Here's how the part is built. I have some questions about the finished solid (model axes, mm). A direction names the side the tool comes from. Give positions to 0.01 mm unless a question says otherwise; leave off trailing zeros. Loops run counter-clockwise (first coordinate to the right, second up) from the corner with the lowest first, then second, coordinate; pieces in that order, holes last. Notation, with made-up numbers: (87.25, 67.25) - (145.25, 67.25) arc R22 ccw to (145.25, 105.25) - close; hole circle Ø6 at (30.5, 54). An arc over 180 degrees is marked (long way). Return JSON: item names as keys, results as strings. Group by question number.
(1) I need wall thicknesses on probe 1 along Y at (x, z) = (50, 2.5); probe 2 along X at (y, z) = (-33, 29); probe 3 along Y at (x, z) = (-183.5, 14.5). Which ranges of each line are inside material? Lowest first, please. Write a range as [from, to].
(2) If we section it at D-D (z = 39.5): State how many separate pieces and enclosed holes the cut face has, then the cut area to 3 significant figures.
(3) If we mould it in two halves opening along X, with no side actions, what happens to faces 1 (the flat face through (204.032, 79, 25)), 2 (the flat face through (-227.768, 30, 25)), 3 (the flat face through (115, 0, 25)), 4 (the flat face through (-2, 81, 0))? For each: released by +X, released by -X, zero draft, split by the parting line, or undercut.
(4) If we section it at A-A (y = -40.5): Please give me the cut outline in (x, z), then the cut area to 3 significant figures.
(5) On a 3-axis mill with a long thin cutter (end or side, diameter ignored), from which of +Z, -Z, +X, -X, +Y, -Y can I reach the whole of each face in a straight line? I mean faces 5 (the flat face through (-2, -201.924, 25)), 6 (the flat face through (-202.368, 78, 25)). Say none if no direction works.
(6) If we section it at B-B (x = 93): Please give me the cut outline in (y, z).
(7) If we section it at C-C (y = 188): Please give me the cut outline in (x, z), then the cut area to 3 significant figures.
```python
from build123d import *

# Parameters (mm, degrees)
F1_DEPTH = 50.8
F2_DEPTH = 50.8
F3_DEPTH = 50.8
F0_W     = 53.3528286101
F0_H     = 176.523585695
F0_W_2   = 176.523585695
F0_H_2   = 53.3528286101
F4_DEPTH = 50.8


with BuildPart() as f1:
    # F0 (on Top) → F1 (new body)
    with BuildSketch(Plane.XY):
        Polygon((-202.3678548309, 229.876414305), (-227.7678548309, 255.276414305), (-227.7678548309, -201.923585695), (-202.3678548309, -176.523585695), (-202.3678548309, -104.6815367264), (-202.3678548309, -50.8), (-202.3678548309, 0), (-202.3678548309, 53.3528286101), (-202.3678548309, 104.1528286101), (-202.3678548309, 158.0343653365), align=None)
        Polygon((-202.3678548309, -176.523585695), (-227.7678548309, -201.923585695), (229.4321451691, -201.923585695), (204.0321451691, -176.523585695), (132.1900962006, -176.523585695), (78.3085594741, -176.523585695), (27.5085594741, -176.523585695), (-25.8442691359, -176.523585695), (-76.6442691359, -176.523585695), (-130.5258058623, -176.523585695), align=None)
        Polygon((229.4321451691, -201.923585695), (229.4321451691, 255.276414305), (204.0321451691, 229.876414305), (204.0321451691, 158.0343653365), (204.0321451691, 104.1528286101), (204.0321451691, 53.3528286101), (204.0321451691, 0), (204.0321451691, -50.8), (204.0321451691, -104.6815367264), (204.0321451691, -176.523585695), align=None)
        Polygon((229.4321451691, 255.276414305), (-227.7678548309, 255.276414305), (-202.3678548309, 229.876414305), (-130.5258058623, 229.876414305), (-76.6442691359, 229.876414305), (-25.8442691359, 229.876414305), (27.5085594741, 229.876414305), (78.3085594741, 229.876414305), (132.1900962006, 229.876414305), (204.0321451691, 229.876414305), align=None)
    extrude(amount=F1_DEPTH)

    # F0 (on Top) → F2 (cut)
    with BuildSketch(Plane.XY):
        Polygon((-76.6442691359, 229.876414305), (-130.5258058623, 229.876414305), (-202.3678548309, 158.0343653365), (-202.3678548309, 104.1528286101), align=None)
    extrude(amount=F2_DEPTH, mode=Mode.SUBTRACT)

    # F0 (on Top) → F3 (join)
    with BuildSketch(Plane.XY):
        Polygon((132.1900962006, -176.523585695), (204.0321451691, -104.6815367264), (204.0321451691, -50.8), (78.3085594741, -176.523585695), align=None)
        Polygon((204.0321451691, 158.0343653365), (132.1900962006, 229.876414305), (78.3085594741, 229.876414305), (204.0321451691, 104.1528286101), align=None)
        Polygon((-76.6442691359, 229.876414305), (-130.5258058623, 229.876414305), (-202.3678548309, 158.0343653365), (-202.3678548309, 104.1528286101), align=None)
        Polygon((-202.3678548309, -104.6815367264), (-130.5258058623, -176.523585695), (-76.6442691359, -176.523585695), (-202.3678548309, -50.8), align=None)
    extrude(amount=F3_DEPTH)

    # F0 (on Top) → F4 (join)
    with BuildSketch(Plane.XY):
        with Locations((0.8321451691, -88.2617928475)):
            Rectangle(F0_W, F0_H)
        with Locations((115.7703523216, 26.676414305)):
            Rectangle(F0_W_2, F0_H_2)
        with Locations((0.8321451691, 141.6146214575)):
            Rectangle(F0_W, F0_H)
        with Locations((-114.1060619834, 26.676414305)):
            Rectangle(F0_W_2, F0_H_2)
        with Locations((0.8321451691, 26.676414305)):
            Rectangle(F0_W, F0_H_2)
    extrude(amount=F4_DEPTH)


solid = f1.part
```
Values:
{
 "1": {"probe 1": "[-201.92, -176.52], [0, 53.35], [229.88, 255.28]", "probe 2": "[-227.77, -202.37], [-25.84, 27.51], [204.03, 229.43]", "probe 3": "[-201.92, -176.52], [-123.55, -69.67], [0, 53.35], [123.02, 176.9], [229.88, 255.28]"},
 "2": {"separate pieces": "1", "enclosed holes": "8", "area": "106,000 mm2"},
 "3": {"face 1": "undercut", "face 2": "released by -X", "face 3": "undercut", "face 4": "zero draft"},
 "4": {"outline": "(-227.77, 0) - (-202.37, 0) - (-202.37, 50.8) - (-227.77, 50.8) - close; (-25.84, 0) - (27.51, 0) - (27.51, 50.8) - (-25.84, 50.8) - close; (204.03, 0) - (229.43, 0) - (229.43, 50.8) - (204.03, 50.8) - close", "area": "5,290 mm2"},
 "5": {"face 5": "+Z, -Z, +X, -X, -Y", "face 6": "+Z, -Z"},
 "6": {"outline": "(-201.92, 0) - (-161.83, 0) - (-161.83, 50.8) - (-201.92, 50.8) - close; (0, 0) - (53.35, 0) - (53.35, 50.8) - (0, 50.8) - close; (215.18, 0) - (255.28, 0) - (255.28, 50.8) - (215.18, 50.8) - close"},
 "7": {"outline": "(-227.77, 0) - (-202.37, 0) - (-202.37, 50.8) - (-227.77, 50.8) - close; (-172.4, 0) - (-118.52, 0) - (-118.52, 50.8) - (-172.4, 50.8) - close; (-25.84, 0) - (27.51, 0) - (27.51, 50.8) - (-25.84, 50.8) - close; (120.18, 0) - (174.07, 0) - (174.07, 50.8) - (120.18, 50.8) - close; (204.03, 0) - (229.43, 0) - (229.43, 50.8) - (204.03, 50.8) - close", "area": "10,800 mm2"}
}
